```python
from build123d import *

# Parameters (mm, degrees)
F1_R = 3.175


with BuildPart() as f2:
    # F2: sweep along a path in F0
    with BuildLine(Plane.XZ) as f2_path:
        Line((-38.1, 698.881), (38.1, 698.881))
        Line((38.1, 698.881), (316.4449418371, 624.2986946097))
        Line((316.4449418371, 624.2986946097), (382.4360776054, 586.1986946097))
        Line((382.4360776054, 586.1986946097), (586.1987574488, 382.4360944431))
        Line((586.1987574488, 382.4360944431), (624.2987574488, 316.4449586747))
        Line((624.2987574488, 316.4449586747), (698.881, 38.1))
        Line((698.881, 38.1), (698.881, -38.1))
        Line((698.881, -38.1), (624.2986946097, -316.4449418371))
        Line((624.2986946097, -316.4449418371), (586.1986946097, -382.4360776054))
        Line((586.1986946097, -382.4360776054), (382.4360944431, -586.1987574488))
        Line((382.4360944431, -586.1987574488), (316.4449586747, -624.2987574488))
        Line((316.4449586747, -624.2987574488), (38.1, -698.881))
        Line((38.1, -698.881), (-38.1, -698.881))
        Line((-38.1, -698.881), (-316.4449418371, -624.2986946097))
        Line((-316.4449418371, -624.2986946097), (-382.4360776054, -586.1986946097))
        Line((-382.4360776054, -586.1986946097), (-586.1987574488, -382.4360944431))
        Line((-586.1987574488, -382.4360944431), (-624.2987574488, -316.4449586747))
        Line((-624.2987574488, -316.4449586747), (-698.881, -38.1))
        Line((-698.881, -38.1), (-698.881, 38.1))
        Line((-698.881, 38.1), (-624.2987574488, 316.4449586747))
        Line((-624.2987574488, 316.4449586747), (-586.1987574488, 382.4360944431))
        Line((-586.1987574488, 382.4360944431), (-382.4360776054, 586.1986946097))
        Line((-382.4360776054, 586.1986946097), (-316.4449418371, 624.2986946097))
        Line((-316.4449418371, 624.2986946097), (-38.1, 698.881))
    # F1 (on Right) → F2 (sweep)
    with BuildSketch(Plane.YZ):
        with Locations((0.9842328243, 701.8995941674)):
            Circle(F1_R)
    sweep(path=f2_path.line, transition=Transition.RIGHT)


solid = f2.part
```
Design review of the part built by this model. Coordinates are the model's own, in mm. Give positions to 0.01 mm unless a question says otherwise; leave off trailing zeros. Order: outer loops, then holes, each group sorted by start corner. A loop starts at its lowest first (then second) coordinate and runs counter-clockwise, first axis right, second up. Notation, with made-up numbers: (-17.5, 44) -> (6.5, 44) arc R33 cw to (6.5, 76) -> close; hole circle Ø9 at (52, -8). An arc over 180 degrees is marked (long way). Write each question's results on one line, items separated by ' | '. Start each with the question number.
Q1. Add section A-A on z = 10.5. Give the boundary of the cut face in (x, y) (3 decimals), and give its area (3 significant figures).
Q2. For pin 1 (3 mm diameter, centred on x = -435.5, y = 0, fed in from +Z); pin 2 (1 mm diameter, centred on y = 3, z = 232, fed in from -X); pin 3 (3 mm diameter, centred on x = 339, y = 3, fed in from -Z), all flat-tipped, find the tip position at first contact; note any pin that passes through.
Q3. Wall thickness on L1, parallel to Z at x = 579.5, y = 3.5; L2, parallel to X at y = -1, z = 314 (3 decimals); L3, parallel to Z at x = -81, y = 1.5: over which ranges is each line inside the solid? List them lowest first. Write a range as from..to.
Found:
1) outline: circle Ø6.35 at (-701.9, 0.984); circle Ø6.35 at (701.9, 0.984) | area: 63.3 mm2
2) pin 1: stops at z = 543.26 | pin 2: stops at x = -652.97 | pin 3: stops at z = -618.89
3) L1: z = -396.14..-390.66, 390.66..396.14 | L2: x = -630.645..-625.513, 625.513..630.645 | L3: z = -693.75..-687.27, 687.27..693.75
